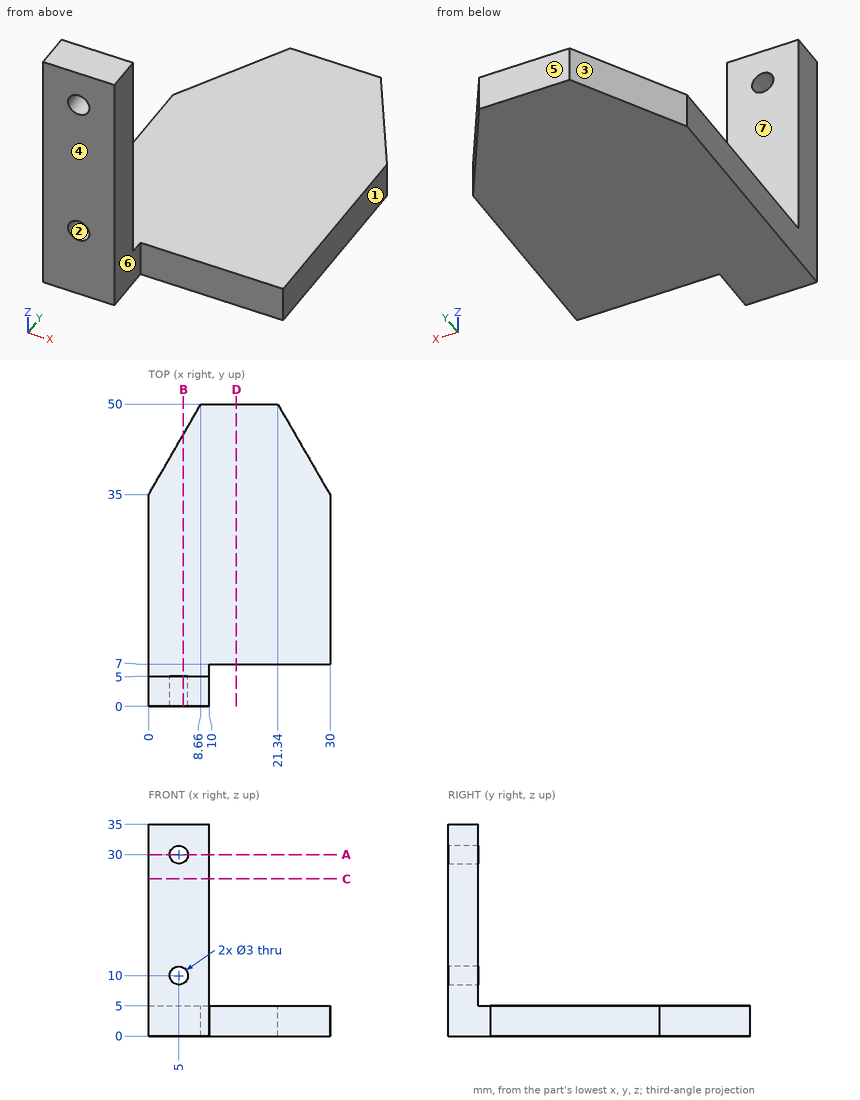
Could you check a few things on this drawing? It's one solid part, dimensions in mm from its lowest x, y, z. A direction names the side the tool comes from. Coordinates: 2 decimals unless noted, no trailing zeros. Order: outer loops, then holes, each group sorted by start corner. A loop starts at its lowest first (then second) coordinate and runs counter-clockwise, first axis right, second up. Notation, with made-up numbers: (62, -27.75) -> (92, -27.75) arc R23 ccw to (92, 1.25) -> close; hole circle Ø11 at (-6.75, 43.5). An arc over 180 degrees is marked (long way). Answer in a Markdown table with one row per item.
(1) On a 3-axis mill with a long thin cutter (end or side, diameter ignored), from which of +Z, -Z, +X, -X, +Y, -Y can I reach the whole of each face in a straight line? I mean the marked faces 5, 6 and 7. Say none if no direction works.
Answer key:
| item | result |
|---|---|
| face 5 | +Z, -Z, +X, -X, +Y |
| face 6 | +Z, -Z, +X, -Y |
| face 7 | +Z, +X, -X, +Y |
(2) I want a section at D-D on x = 14.5. List the corners of the cut face in (y, z) for me, then the cut area to 3 significant figures.
Answer key:
| item | result |
|---|---|
| outline | (7, 0) -> (50, 0) -> (50, 5) -> (7, 5) -> close |
| area | 215 mm^2 |
(3) I want a section at B-B on x = 5.75. List the corners of the cut face in (y, z) for me, then the cut area to 3 significant figures.
Answer key:
| item | result |
|---|---|
| outline | (0, 0) -> (44.96, 0) -> (44.96, 5) -> (5, 5) -> (5, 8.7) -> (0, 8.7) -> close; (0, 11.3) -> (5, 11.3) -> (5, 28.7) -> (0, 28.7) -> close; (0, 31.3) -> (5, 31.3) -> (5, 35) -> (0, 35) -> close |
| area | 349 mm^2 |
(4) I want a section at C-C on z = 26. List the corners of the cut face in (x, y) for me.
Answer key:
| item | result |
|---|---|
| outline | (0, 0) -> (10, 0) -> (10, 5) -> (0, 5) -> close |
(5) Please list where these lines run through material, in increasing order: probe 1 along X at (y, z) = (2.55, 30); probe 2 along Y at (x, z) = (2.5, 22).
Answer key:
| item | result |
|---|---|
| probe 1 | 0 to 3.5, 6.5 to 10 |
| probe 2 | 0 to 5 |
(6) Thinking about a two-plate mould opening in X: for the marked faces 1, 2, 3 and 4, which applies, +X half, -X half, draft (parallel to the pull), parting line (faces both ways), or undercut?
Answer key:
| item | result |
|---|---|
| face 1 | +X half |
| face 2 | undercut |
| face 3 | -X half |
| face 4 | draft |
(7) Will these pins go through, and if not, where does the flat tip stop? pin 1 Ø8 at (x, z) = (5, 16.5) entering from +Y; pin 2 Ø2 at (x, z) = (24.5, 6.5) entering from +Y; pin 3 Ø2 at (y, z) = (2, 16.5) entering from +X; pin 4 Ø1.5 at (x, z) = (21.5, 3) entering from -Y.
Answer key:
| item | result |
|---|---|
| pin 1 | y = 5 |
| pin 2 | through |
| pin 3 | x = 10 |
| pin 4 | y = 7 |
(8) I want a section at A-A on z = 30. List the corners of the cut face in (x, y) for me, then the cut area to 3 significant figures.
Answer key:
| item | result |
|---|---|
| outline | (0, 0) -> (3.5, 0) -> (3.5, 5) -> (0, 5) -> close; (6.5, 0) -> (10, 0) -> (10, 5) -> (6.5, 5) -> close |
| area | 35.0 mm^2 |
